Here's how the part is built. I have some questions about the finished solid (model axes, mm). A direction names the side the tool comes from. Coordinates: 2 decimals unless noted, no trailing zeros. Loops run counter-clockwise (first coordinate to the right, second up) from the corner with the lowest first, then second, coordinate; pieces in that order, holes last.
Autodesk Inventor part; units mm, degrees
ref_plane "YZ Plane" through (0, 0, 0) normal (1, 0, 0) x (0, 1, 0)
ref_plane "XZ Plane" through (0, 0, 0) normal (0, 1, 0) x (-1, 0, 0)
ref_plane "XY Plane" through (0, 0, 0) normal (0, 0, 1) x (1, 0, 0)
sketch "Sketch1" plane through (0, 0, 0) normal (1, 0, 0) x (0, 1, 0)
  line L0 (0, 0) -> (32.5, 0)
  line L1 (32.5, 0) -> (32.5, -13)
  line L2 (32.5, -60) -> (0, -60)
  line L3 (0, -60) -> (0, 0)
  circle A0 centre (22, -53) radius 3.3
  circle A1 centre (22, -7) radius 3.3
  circle A2 centre (7, -7) radius 3.3
  circle A3 centre (7, -53) radius 3.3
  line L4 (22, -7) -> (7, -7) construction
  line L5 (7, -7) -> (7, -53) construction
  line L6 (7, -53) -> (22, -53) construction
  line L7 (22, -53) -> (22, -7) construction
  line L8 (32.5, -13) -> (39, -13)
  line L9 (39, -13) -> (39, -47)
  line L10 (39, -47) -> (32.5, -47)
  line L11 (32.5, -47) -> (32.5, -60)
  line L12 (32.5, -13) -> (32.5, -47) construction
  circle A4 centre (22, -30) radius 5
  point P0 (32.5, -30)
  dimension "d0" = 60
  dimension "d1" = 6.6
  dimension "d2" = 15
  dimension "d3" = 46
  dimension "d4" = 22
  dimension "d5" = 32.5
  dimension "d6" = 34
  dimension "d7" = 39
  dimension "d8" = 10
extrude "Extrusion1" add sketch "Sketch1" along normal blind 25
sketch "Sketch2" plane through (25, 0, 0) normal (1, 0, 0) x (0, 0, -1)
  line L0 (47, 39) -> (13, 39)
  line L1 (13, 39) -> (13, 5)
  line L2 (13, 5) -> (47, 5)
  line L3 (47, 5) -> (47, 39)
  circle A0 centre (30, 22) radius 5
  point P0 (0, 0)
extrude "Extrusion2" add sketch "Sketch2" along normal blind 5
sketch "Sketch3" plane through (30, 0, 0) normal (1, 0, 0) x (0, 0, -1)
  circle A0 centre (30, 22) radius 5
  circle A1 centre (30, 22) radius 5
  line L0 (20.1863, 23.5) -> (20.1863, 20.5)
  line L1 (20.1863, 20.5) -> (28.5, 12.1863)
  line L2 (28.5, 12.1863) -> (31.5, 12.1863)
  line L3 (31.5, 12.1863) -> (39.8137, 20.5)
  line L4 (39.8137, 20.5) -> (39.8137, 23.5)
  line L5 (39.8137, 23.5) -> (31.5, 31.8137)
  line L6 (31.5, 31.8137) -> (28.5, 31.8137)
  line L7 (28.5, 31.8137) -> (20.1863, 23.5)
  point P0 (0, 0)
  point P1 (30, 12.1863)
  point P2 (20.1863, 22)
  point P3 (35.6569, 27.6569)
  point P4 (24.3431, 16.3431)
  dimension "d14" = 135
  dimension "d15" = 16
  dimension "d16" = 3
extrude "Extrusion3" add sketch "Sketch3" along normal blind 4.5
sketch "Sketch4" plane through (0, 32.5, -47) normal (0, 1, 0) x (1, 0, 0)
  circle A0 centre (6, -40) radius 5.4
  point P0 (0, -47)
  dimension "d19" = 10.8
  dimension "d20" = 6
  dimension "d21" = 7
extrude "Extrusion4" cut sketch "Sketch4" against normal blind 5
sketch "Sketch5" plane through (6, 27.5, -7) normal (0, 1, 0) x (1, 0, 0)
  circle A0 centre (0, 0) radius 3.3
  circle A1 centre (0, 0) radius 5.4 construction
  point P0 (-6, -7)
  dimension "d24" = 6.6
extrude "Extrusion5" cut sketch "Sketch5" against normal up to surface (27.5 mm away)
pattern_linear "Rectangular Pattern1" count 2 spacing 13 along (1, 0, 0) count 2 spacing -46 along (0, 0, 1) of "Extrusion5", "Extrusion4"
properties part number "BK10_Frame"
Q1. We'd pull the mould along Y, two halves only. Please class faces 1 (the cylindrical face through (2.29, 21.28, -3.78)), 2 (the flat face through (12, 0, -30)), 3 (the flat face through (12, 32.5, -6)), 4 (the flat face through (19, 33, -13)): pulls with the +Y half, pulls with the -Y half, needs draft (parallel to the pull), parting line crosses it, or undercut.
Q2. For faces 5 (the flat face through (32, 31.814, -30)), 6 (the flat face through (32, 22, -20.186)), 7 (the cylindrical face through (1.715, 30.035, -3.714)), which set-ups out of +Z, -Z, +X, -X, +Y, -Y let a thin tool reach every point of the face, with its end or its side?
Q3. Suppose I cut it at B-B on z = -27.5. Write out the boundary of the cut face in (x, y).
Q4. Suppose I cut it at C-C on x = 32. Write out the boundary of the cut face in (y, z), and give its area (3 significant figures).
Q5. Will these pins go through, and if not, where does the flat tip stop? P1, Ø0.9, axis at x = 31.5, z = -29.5, coming from the +Y side; P2, Ø3, axis at x = 6.5, y = 5.5, coming from the +Z side; P3, Ø0.9, axis at x = 32, y = 21.5, coming from the +Z side; P4, Ø3, axis at y = 26, z = -47, coming from the +X side.
Q6. Please list where these lines run through material, in increasing order: probe 1 along Z at (x, y) = (22.25, 7); probe 2 along Y at (x, z) = (23, -30); probe 3 along Z at (x, y) = (13, 9.5).
Q7. Suppose I cut it at D-D on z = -53. State how many separate pieces and enclosed holes the cut face has, and give its area (3 significant figures).
Q8. Suppose I cut it at A-A on x = 12.5. Write out the boundary of the cut face in (y, z).
Check values:
1. face 1: undercut
1. face 2: pulls with the -Y half
1. face 3: pulls with the +Y half
1. face 4: needs draft
2. face 5: +Z, -Z, +X, +Y
2. face 6: +Z, +X, +Y, -Y
2. face 7: +Y
3. outline: (0, 0) - (25, 0) - (25, 5) - (30, 5) - (30, 13.19) - (34.5, 13.19) - (34.5, 17.67) - (0, 17.67) - close; (0, 26.33) - (34.5, 26.33) - (34.5, 30.81) - (30, 30.81) - (30, 39) - (0, 39) - close
4. outline: (12.19, -31.5) - (20.5, -39.81) - (23.5, -39.81) - (31.81, -31.5) - (31.81, -28.5) - (23.5, -20.19) - (20.5, -20.19) - (12.19, -28.5) - close; hole circle Ø10 at (22, -30)
4. area: 168 mm2
5. P1: stops at y = 31.81
5. P2: stops at z = 0
5. P3: stops at z = -20.19
5. P4: stops at x = 30
6. probe 1: z = -60 to -56.3, -49.7 to -10.3, -3.7 to 0
6. probe 2: y = 0 to 17, 27 to 39
6. probe 3: z = -60 to -55.15, -50.85 to -9.15, -4.85 to 0
7. separate pieces: 9
7. enclosed holes: 0
7. area: 186 mm2
8. outline: (0, -60) - (32.5, -60) - (32.5, -47) - (39, -47) - (39, -13) - (32.5, -13) - (32.5, 0) - (0, 0) - close; hole circle Ø6.6 at (7, -53); hole circle Ø6.6 at (7, -7); hole circle Ø10 at (22, -30); hole circle Ø6.6 at (22, -53); hole circle Ø6.6 at (22, -7)
